```python
from build123d import *

# Parameters (mm, degrees)
F0_R     = 25
F1_DEPTH = 10
F5_W     = 20
F5_H     = 20
F6_DEPTH = 31
F7_SIZE  = 1
F8_R     = 5
F9_R     = 2


# Not quite as in the source:
# - a feature names something its author has since deleted; it is built from what else it names


with BuildPart() as f1:
    # F0 (on Right) → F1 (new body)
    with BuildSketch(Plane.YZ):
        Circle(F0_R)
    extrude(amount=F1_DEPTH)

    # F5 (on offset) → F6 (join)
    with BuildSketch(Plane(origin=(6.9318764812, 0.9742117067, 0), x_dir=(0.139173101, -0.9902680687, 0), z_dir=(-0.9902680687, -0.139173101, 0))):
        Rectangle(F5_W, F5_H)
    extrude(amount=-F6_DEPTH)

    # F7
    f7_edges = [f1.edges().sort_by_distance(p)[0] for p in [
        (39.021918, -4.614103, 0),
        (37.630187, 5.288578, 10),
        (36.238456, 15.191259, 0),
        (37.630187, 5.288578, -10),
    ]]
    chamfer(f7_edges, length=F7_SIZE)

    # F8
    f8_edges = [f1.edges().sort_by_distance(p)[0] for p in [
        (10, -25, 0),
    ]]
    fillet(f8_edges, radius=F8_R)

    # F9
    f9_edges = [f1.edges().sort_by_distance(p)[0] for p in [
        (10, 1.405408, -10),
        (10, -8.692867, 0),
        (10, 1.405408, 10),
        (10, 11.503684, 0),
    ]]
    fillet(f9_edges, radius=F9_R)


solid = f1.part
```
Could you check a few things on this model? Use its own coordinates, in mm. A direction names the side the tool comes from. Round coordinates to 2 decimals unless told otherwise and drop trailing zeros. Write each loop counter-clockwise with the first axis right and the second up, starting at its lowest first coordinate (ties: lowest second). Pieces come first, ordered by that corner, then holes. Notation, with made-up numbers: M 15.5,-1 L 67.5,-1 A16 cw 67.5,11 Z; hole C 28,17.25 d2. An arc over 180 degrees is marked long. Write each question's results on one line, items separated by ' | '. Start each with the question number.
1. Imagine slicing it at D-D on x = 23.5. List the corners of the cut face in (y, z) for me, and give its area (3 significant figures).
2. Imagine slicing it at B-B on x = 3. List the corners of the cut face in (y, z) for me, and give its area (3 significant figures).
3. Imagine slicing it at A-A on z = 0. List the corners of the cut face in (x, y) for me, and give its area (3 significant figures).
4. I'm going to push flat-ended pins straight in: pin 1 Ø3 at (x, y) = (34, -3) entering from +Z; pin 2 Ø19 at (x, y) = (22.5, 5.5) entering from -Z; pin 3 Ø10 at (y, z) = (-7, 9) entering from -X; pin 4 Ø4 at (x, y) = (4, 10) entering from -Z. Where does each tip first touch, or does it pass through?
5. Thinking about a two-plate mould opening in X: for faces 1 (the face through (10.48, -9.13, -0.17)), 2 (the face through (2.465, 23.846, 7.509)), 3 (the face through (23.602, 13.415, -0.14)), which applies, +X half, -X half, draft (parallel to the pull), parting line (faces both ways), or undercut?
6. On a 3-axis mill with a long thin cutter (end or side, diameter ignored), from which of +Z, -Z, +X, -X, +Y, -Y can I reach the whole of each face in a straight line? I mean faces 4 (the face through (23, 3, 10)), 5 (the face through (37.123, 5.359, 9.493)), 6 (the face through (23, 3, -10)). Say none if no direction works.
7. I need wall thicknesses on L1, parallel to X at y = -7, z = -18; L2, parallel to Z at x = 15, y = 7; L3, parallel to Y at x = 18, z = 8. Which ranges of each line are inside material? Lowest first, please. Write a range as from..to.
8. Imagine slicing it at C-C on y = 0. List the corners of the cut face in (x, z) for me, and give its area (3 significant figures).
Result sheet:
1) outline: M -6.8,-10 L 13.4,-10 L 13.4,10 L -6.8,10 Z | area: 404 mm^2
2) outline: C 0,0 d50 | area: 1,960 mm^2
3) outline: M 0,-25 L 5,-25 A5 ccw 10,-20 L 10,-10.43 A2 cw 11.72,-8.45 L 38.03,-4.75 L 38.88,-3.62 L 36.38,14.2 L 35.25,15.05 L 12.28,11.82 A2 cw 10,13.8 L 10,20 A5 ccw 5,25 L 0,25 Z | area: 1,050 mm^2
4) pin 1: stops at z = 10 | pin 2: stops at z = -10 | pin 3: stops at x = 0 | pin 4: stops at z = -23.69
5) face 1: +X half | face 2: draft | face 3: undercut
6) face 4: +Z, +X, +Y, -Y | face 5: +Z, +X, +Y | face 6: -Z, +X, +Y, -Y
7) L1: x = 0..10 | L2: z = -10..10 | L3: y = -7.57..12.63
8) outline: M 0,-25 L 5,-25 A5 ccw 10,-20 L 10,-12 A2 cw 12,-10 L 37.36,-10 L 38.37,-9 L 38.37,9 L 37.36,10 L 12,10 A2 cw 10,12 L 10,20 A5 ccw 5,25 L 0,25 Z | area: 1,060 mm^2
